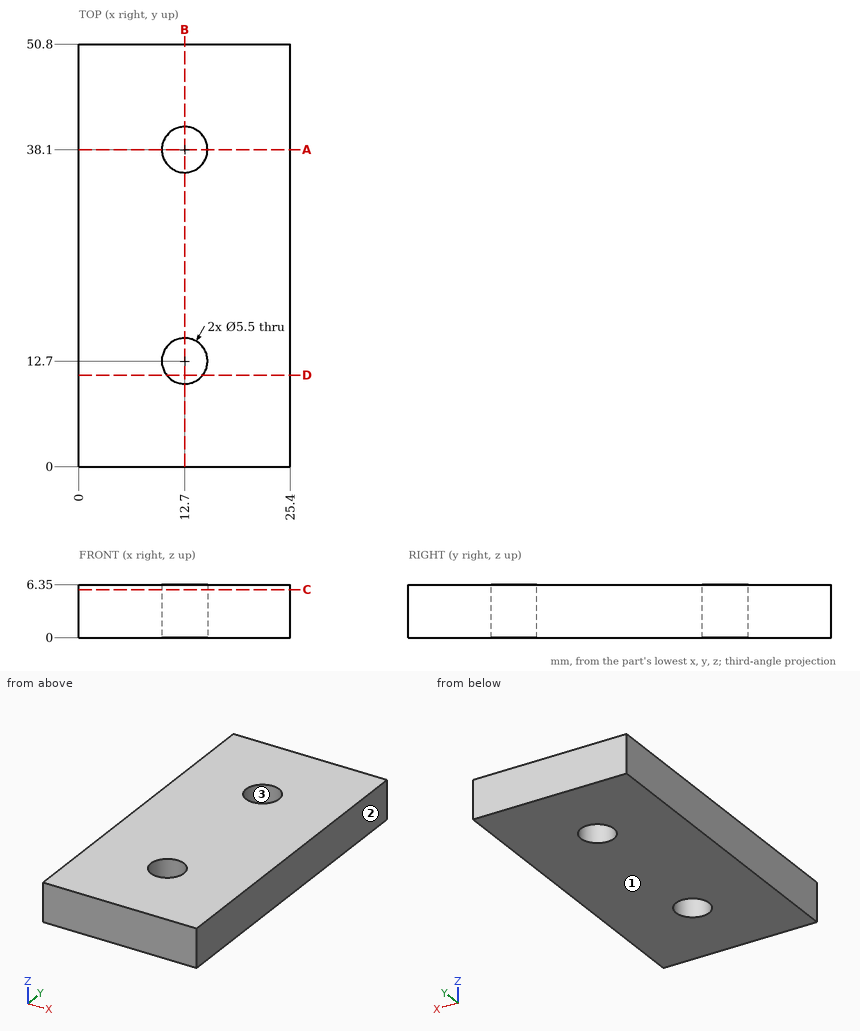
The figure shows three views and two pictorial views of one solid part (mm, origin at its lowest corner). Answer the questions. Coordinates: 2 decimals unless noted, no trailing zeros. Order: outer loops, then holes, each group sorted by start corner. A loop starts at its lowest first (then second) coordinate and runs counter-clockwise, first axis right, second up.
Q1. Consider line 1 (Y direction, x = 12.7, z = 2.5); line 2 (X direction, y = 12.7, z = 3); line 3 (X direction, y = 11.5, z = 3.75). Determine where each line is inside the solid, lowest interval first.
Q2. A cutting plane is placed at B-B, the plane x = 12.7. Write down the section's boundary in (y, z).
Q3. A cutting plane is placed at D-D, the plane y = 11. Write down the section's boundary in (x, z).
Q4. For a pull along X with two mould halves and no side action, classify the marked faces 1, 2 and 3 as pulls with the +X half, pulls with the -X half, needs draft (parallel to the pull), parting line crosses it, or undercut.
Q5. A cutting plane is placed at C-C, the plane z = 5.75. Write down the section's boundary in (x, y), and give its area (3 significant figures).
Q6. A cutting plane is placed at A-A, the plane y = 38.1. Write down the section's boundary in (x, z), and give its area (3 significant figures).
Answers follow:
1. line 1: y = 0 to 9.95, 15.45 to 35.35, 40.85 to 50.8
1. line 2: x = 0 to 9.95, 15.45 to 25.4
1. line 3: x = 0 to 10.23, 15.17 to 25.4
2. outline: (0, 0) - (9.95, 0) - (9.95, 6.35) - (0, 6.35) - close; (15.45, 0) - (35.35, 0) - (35.35, 6.35) - (15.45, 6.35) - close; (40.85, 0) - (50.8, 0) - (50.8, 6.35) - (40.85, 6.35) - close
3. outline: (0, 0) - (10.54, 0) - (10.54, 6.35) - (0, 6.35) - close; (14.86, 0) - (25.4, 0) - (25.4, 6.35) - (14.86, 6.35) - close
4. face 1: needs draft
4. face 2: pulls with the +X half
4. face 3: undercut
5. outline: (0, 0) - (25.4, 0) - (25.4, 50.8) - (0, 50.8) - close; hole circle Ø5.5 at (12.7, 12.7); hole circle Ø5.5 at (12.7, 38.1)
5. area: 1,240 mm2
6. outline: (0, 0) - (9.95, 0) - (9.95, 6.35) - (0, 6.35) - close; (15.45, 0) - (25.4, 0) - (25.4, 6.35) - (15.45, 6.35) - close
6. area: 126 mm2
